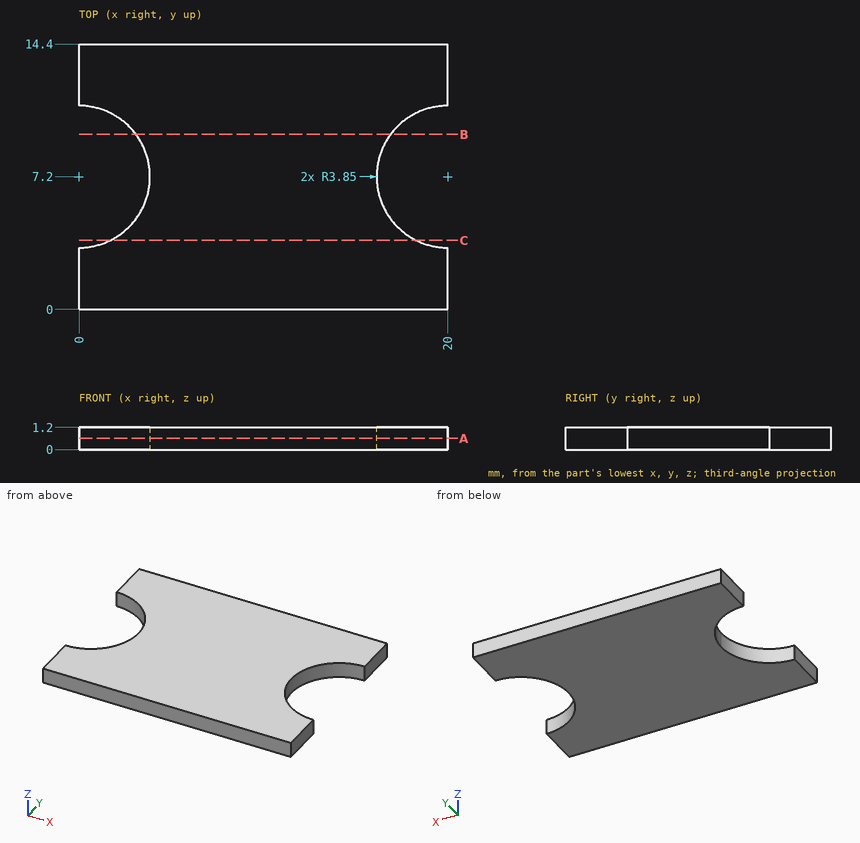
Here's the drawing with two shaded views (mm, measured from the low corner). I have some questions. Give positions to 0.01 mm unless a question says otherwise; leave off trailing zeros. Loops run counter-clockwise (first coordinate to the right, second up) from the corner with the lowest first, then second, coordinate; pieces in that order, holes last. Notation, with made-up numbers: M 71.5,-24 L 101.5,-24 A15 ccw 101.5,-13 Z; hole C 41,27.5 d8. An arc over 180 degrees is marked long. One line per item, written item: value. Start each with the question number.
1) If we section it at C-C, the plane y = 3.75: Write out the boundary of the cut face in (x, z), and give its area (3 significant figures).
2) If we section it at A-A, the plane z = 0.6: Write out the boundary of the cut face in (x, y), and give its area (3 significant figures).
3) If we section it at B-B, the plane y = 9.5: Write out the boundary of the cut face in (x, z).
4) If I drill on line 1 (Y direction, x = 17.5, z = 0.8); line 2 (Y direction, x = 19, z = 1); line 3 (X direction, y = 7.5, z = 0.8), over which ranges is the centre line in solid material (lowest first)? Write a range as [from, to].
Completed:
1. outline: M 1.71,0 L 18.29,0 L 18.29,1.2 L 1.71,1.2 Z
1. area: 19.9 mm^2
2. outline: M 0,0 L 20,0 L 20,3.35 A3.85 cw 20,11.05 L 20,14.4 L 0,14.4 L 0,11.05 A3.85 cw 0,3.35 Z
2. area: 241 mm^2
3. outline: M 3.09,0 L 16.91,0 L 16.91,1.2 L 3.09,1.2 Z
4. line 1: y = [0, 4.27], [10.13, 14.4]
4. line 2: y = [0, 3.48], [10.92, 14.4]
4. line 3: x = [3.84, 16.16]
